The model under review builds one solid part; all positions refer to its coordinate system, in mm. A direction names the side the tool comes from. Coordinates: 2 decimals unless noted, no trailing zeros. Write each loop counter-clockwise with the first axis right and the second up, starting at its lowest first coordinate (ties: lowest second). Pieces come first, ordered by that corner, then holes. Notation, with made-up numbers: (47, 43.25) -> (55, 43.25) arc R25 ccw to (55, 82.25) -> close; hole circle Ø11 at (13, -25.5). An arc over 180 degrees is marked (long way). Write each question's results on one line, items separated by ' | '.
```python
from build123d import *

# Parameters (mm, degrees)
F0_W      = 304.8
F0_H      = 50.8
F1_DEPTH  = 88.9
F2_W      = 304.8
F2_H      = 19.05
F3_DEPTH  = 12.7
F5_DEPTH  = 88.9
F7_DEPTH  = 12.7
F9_DEPTH  = 88.9
F11_DEPTH = 12.7
F13_DEPTH = 12.7


with BuildPart() as f1:
    # F0 (on Top) → F1 (new body)
    with BuildSketch(Plane.XY):
        Rectangle(F0_W, F0_H)
    extrude(amount=F1_DEPTH)

    # F2 (on face) → F3 (cut)
    with BuildSketch(Plane.XY.offset(88.9)):
        with Locations((0, -15.875)):
            Rectangle(F2_W, F2_H)
    extrude(amount=-F3_DEPTH, mode=Mode.SUBTRACT)

    # F4 (on Top) → F5 (join)
    with BuildSketch(Plane.XY):
        Polygon((152.4, 25.4), (152.4, -25.4), (203.2, 25.4), align=None)
    extrude(amount=F5_DEPTH)

    # F6 (on face) → F7 (cut)
    with BuildSketch(Plane.XY.offset(88.9)):
        Polygon((171.45, -6.35), (152.4, -6.35), (152.4, -25.4), align=None)
    extrude(amount=-F7_DEPTH, mode=Mode.SUBTRACT)

    # F8 (on Top) → F9 (join)
    with BuildSketch(Plane.XY):
        Polygon((-203.2, 25.4), (-152.4, -25.4), (-152.4, 25.4), align=None)
    extrude(amount=F9_DEPTH)

    # F10 (on face) → F11 (cut)
    with BuildSketch(Plane.XY.offset(88.9)):
        Polygon((-171.45, -6.35), (-152.4, -25.4), (-152.4, -6.35), align=None)
    extrude(amount=-F11_DEPTH, mode=Mode.SUBTRACT)

    # F12 (on face) → F13 (cut)
    with BuildSketch(Plane(origin=(0, 0, 0), x_dir=(1, 0, 0), z_dir=(0, 0, -1))):
        Polygon((-165.870384, 11.929616), (165.870384, 11.929616), (152.4, 25.4), (-152.4, 25.4), align=None)
    extrude(amount=-F13_DEPTH, mode=Mode.SUBTRACT)


solid = f1.part
```
Q1. For line 1 (Z direction, x = 60.5, y = -7); line 2 (X direction, y = -12, z = 52); line 3 (Z direction, x = -28, y = -18), list the stretches that pass through material, from the lowest coordinate up. Write a range as from..to.
Solution:
line 1: 0..76.2 | line 2: -165.8..165.8 | line 3: 12.7..76.2
Q2. Machinability: for faces 1 (the flat face through (177.4, -0.4, 43.8)), 2 (the flat face through (2, -6.35, 83)), 3 (the flat face through (-2, -19, 12.7)), which of the approach directions +Z, -Z, +X, -X, +Y, -Y give a long, thin tool a straight path to every point of the face, cutting with its end or side? Answer none if there is none.
Solution:
face 1: +Z, -Z, +X, -Y | face 2: +Z, +X, -X, -Y | face 3: -Z, +X, -X, -Y
Q3. Clearance check with flat-ended pins moving along their axes: P1, Ø9.5, axis at x = 66, y = -12.5, coming from the +Z side; P2, Ø8, axis at x = 98.5, y = 2, coming from the -Z side; P3, Ø2, axis at y = 9, z = 25.5, coming from the -X side; P4, Ø10, axis at y = -3.5, z = 42, coming from the +X side. State where each tip first meets the part, or that it passes through.
Solution:
P1: z = 76.2 | P2: z = 0 | P3: x = -187.8 | P4: x = 179.3
Q4. Add section B-B (z = 19.5). Write out the cut boundary in (x, y).
Solution:
outline: (-203.2, 25.4) -> (-152.4, -25.4) -> (152.4, -25.4) -> (203.2, 25.4) -> close
Q5. Add section A-A (x = 13). Write out the cut boundary in (y, z), plus the area to 3 significant figures.
Solution:
outline: (-25.4, 12.7) -> (-11.93, 12.7) -> (-11.93, 0) -> (25.4, 0) -> (25.4, 88.9) -> (-6.35, 88.9) -> (-6.35, 76.2) -> (-25.4, 76.2) -> close | area: 4,100 mm²
Q6. Add section C-C (y = -0.5). Write out the cut boundary in (x, z), plus the area to 3 significant figures.
Solution:
outline: (-177.3, 0) -> (177.3, 0) -> (177.3, 88.9) -> (-177.3, 88.9) -> close | area: 31,500 mm²
